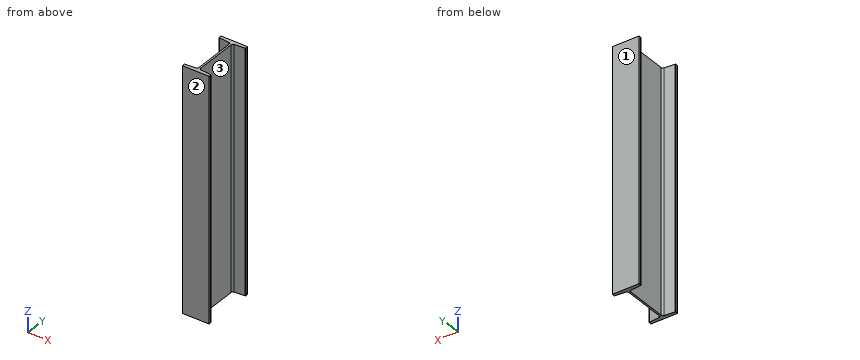
```python
from build123d import *

# Parameters (mm, degrees)
BOSS_EXTRUDE1_START = -457.2
BOSS_EXTRUDE1_DEPTH = 914.4


with BuildPart() as part:
    # Sketch3 → Boss-Extrude1 (new body)
    with BuildSketch(Plane.XY.offset(BOSS_EXTRUDE1_START)):
        with BuildLine():
            Line((-50.8, -101.6), (50.8, -101.6))
            Line((50.8, -101.6), (50.8, -92.783359005))
            ThreePointArc((50.8, -92.783359005), (50.23278177, -91.324759746), (48.829169249, -90.632574652))
            Line((48.829169249, -90.632574652), (9.72517216, -87.211418208))
            ThreePointArc((9.72517216, -87.211418208), (5.25012518, -85.004569258), (3.4417, -80.354211623))
            Line((3.4417, -80.354211623), (3.4417, 80.354211623))
            ThreePointArc((3.4417, 80.354211623), (5.25012518, 85.004569258), (9.72517216, 87.211418208))
            Line((9.72517216, 87.211418208), (48.829169249, 90.632574652))
            ThreePointArc((48.829169249, 90.632574652), (50.23278177, 91.324759746), (50.8, 92.783359005))
            Line((50.8, 92.783359005), (50.8, 101.6))
            Line((50.8, 101.6), (-50.8, 101.6))
            Line((-50.8, 101.6), (-50.8, 92.783359005))
            ThreePointArc((-50.8, 92.783359005), (-50.23278177, 91.324759746), (-48.829169249, 90.632574652))
            Line((-48.829169249, 90.632574652), (-9.72517216, 87.211418208))
            ThreePointArc((-9.72517216, 87.211418208), (-5.25012518, 85.004569258), (-3.4417, 80.354211623))
            Line((-3.4417, 80.354211623), (-3.4417, -80.354211623))
            ThreePointArc((-3.4417, -80.354211623), (-5.25012518, -85.004569258), (-9.72517216, -87.211418208))
            Line((-9.72517216, -87.211418208), (-48.829169249, -90.632574652))
            ThreePointArc((-48.829169249, -90.632574652), (-50.23278177, -91.324759746), (-50.8, -92.783359005))
            Line((-50.8, -92.783359005), (-50.8, -101.6))
        make_face()
    extrude(amount=BOSS_EXTRUDE1_DEPTH)


solid = part.part
```
For this review, take the finished solid that the model builds, in its own axes (mm). Face numbers are marked on the shaded views. Coordinates: 2 decimals unless noted, no trailing zeros. Loops run counter-clockwise (first coordinate to the right, second up) from the corner with the lowest first, then second, coordinate; pieces in that order, holes last.
1. Add section D-D, the plane y = 41. Give the boundary of the cut face in (x, z).
2. Add section C-C, the plane x = -39. Give the boundary of the cut face in (y, z), then the cut area to 3 significant figures.
3. For line 1 (Y direction, x = -10.5, z = -22); line 2 (X direction, y = -19, z = 195.5); line 3 (Y direction, x = 44.5, z = 312.5), list the stretches that pass through material, from the lowest coordinate up.
4. Add section A-A, the plane x = 38. Give the boundary of the cut face in (y, z).
5. Mouldability with a two-part tool opening along Y and no side actions: class the marked faces 1, 2 and 3 as +Y half, -Y half, draft (parallel to the pull), parting line (faces both ways), or undercut.
6. Add section B-B, the plane z = -240. Give the boundary of the cut face in (x, y), then the cut area to 3 significant figures.
Result:
1. outline: (-3.44, -457.2) - (3.44, -457.2) - (3.44, 457.2) - (-3.44, 457.2) - close
2. outline: (-101.6, -457.2) - (-89.77, -457.2) - (-89.77, 457.2) - (-101.6, 457.2) - close; (89.77, -457.2) - (101.6, -457.2) - (101.6, 457.2) - (89.77, 457.2) - close
2. area: 21,600 mm2
3. line 1: y = -101.6 to -87.28, 87.28 to 101.6
3. line 2: x = -3.44 to 3.44
3. line 3: y = -101.6 to -90.25, 90.25 to 101.6
4. outline: (-101.6, -457.2) - (-89.69, -457.2) - (-89.69, 457.2) - (-101.6, 457.2) - close; (89.69, -457.2) - (101.6, -457.2) - (101.6, 457.2) - (89.69, 457.2) - close
5. face 1: +Y half
5. face 2: -Y half
5. face 3: undercut
6. outline: (-50.8, -101.6) - (50.8, -101.6) - (50.8, -92.78) arc R2.16 ccw to (48.83, -90.63) - (9.73, -87.21) arc R6.88 cw to (3.44, -80.35) - (3.44, 80.35) arc R6.88 cw to (9.73, 87.21) - (48.83, 90.63) arc R2.16 ccw to (50.8, 92.78) - (50.8, 101.6) - (-50.8, 101.6) - (-50.8, 92.78) arc R2.16 ccw to (-48.83, 90.63) - (-9.73, 87.21) arc R6.88 cw to (-3.44, 80.35) - (-3.44, -80.35) arc R6.88 cw to (-9.73, -87.21) - (-48.83, -90.63) arc R2.16 ccw to (-50.8, -92.78) - close
6. area: 3,870 mm2
